```python
from build123d import *

# Parameters (mm, degrees)
F0_W           = 40.7
F0_H           = 23.2
F0_H_2         = 5
F0_H_3         = 1.8
F1_DEPTH       = 10.5
F2_D           = 3
F2_CBORE_D     = 6
F2_CBORE_DEPTH = 5
F3_D           = 3
F3_CBORE_D     = 6
F3_CBORE_DEPTH = 5
F4_DEPTH       = 4
F6_DEPTH       = 8.8
F7_T1_DEPTH    = 13.8
F7_T3_DEPTH    = 20.5
F7_T5_DEPTH    = 33.2
F7_T7_DEPTH    = 50.6498743711
F7_T9_DEPTH    = 50.7
F7_T11_DEPTH   = 5
F8_R           = 0.5
F10_DEPTH      = 2.5
F11_DEPTH      = 1.5


# Not quite as in the source:
# - a fillet or chamfer that OpenCascade refuses, or shapes differently, is made with other operations: its cross-section is extruded or revolved along the edge and cut away or added


with BuildPart() as f1:
    # F0 (on Top) → F1 (new body)
    with BuildSketch(Plane.XY):
        with Locations((0, -3.4)):
            Rectangle(F0_W, F0_H)
        with Locations((0, 10.7)):
            Rectangle(F0_W, F0_H_2)
        with Locations((0, 14.1)):
            Rectangle(F0_W, F0_H_3)
    extrude(amount=F1_DEPTH)

    # F2 (through all)
    with Locations(Plane(origin=(0, 0, 0), x_dir=(1, 0, 0), z_dir=(0, 0, -1))):
        with Locations((-16.15, 10.5)):
            CounterBoreHole(F2_D / 2, F2_CBORE_D / 2, F2_CBORE_DEPTH)

    # F3 (through all)
    with Locations(Plane(origin=(0, 0, 0), x_dir=(1, 0, 0), z_dir=(0, 0, -1))):
        with Locations((16.15, 10.5)):
            CounterBoreHole(F3_D / 2, F3_CBORE_D / 2, F3_CBORE_DEPTH)

    # F0 (on Top) → F4 (cut)
    with BuildSketch(Plane.XY):
        with Locations((0, 10.7)):
            Rectangle(F0_W, F0_H_2)
    extrude(amount=F4_DEPTH, mode=Mode.SUBTRACT)

    # F5 (on face) → F6 (cut)
    with BuildSketch(Plane.XY.offset(10.5)):
        Polygon((-12.85, -3.7), (-12.85, -8.6720474064), (-12.85, -15), (12.85, -15), (12.85, -8.5788490251), (12.886153895, -3.7037077804), (14.5, -3.7156760127), (14.5, 8.1671951339), (-14.5, 8.0755921081), (-14.5, -3.7), align=None)
    extrude(amount=-F6_DEPTH, mode=Mode.SUBTRACT)

    # F7: fillet of radius 2 on 10 edges, made by hand

    # F7_s2 → F7_t1 (cut)
    with BuildSketch(Plane.XY.offset(1.7)):
        with BuildLine():
            ThreePointArc((-14.85, -15), (-13.4357864376, -14.4142135624), (-12.85, -13))
            Line((-12.85, -13), (-12.85, -15))
            Line((-12.85, -15), (-14.85, -15))
        make_face()
        with BuildLine():
            ThreePointArc((14.85, -15), (13.4357864376, -14.4142135624), (12.85, -13))
            Line((12.85, -13), (12.85, -15))
            Line((12.85, -15), (14.85, -15))
        make_face()
    extrude(amount=F7_T1_DEPTH, mode=Mode.SUBTRACT)

    # F7_s4 → F7_t3 (cut)
    with BuildSketch(Plane.XY.offset(-5)):
        with BuildLine():
            ThreePointArc((-18.35, -15), (-19.7642135624, -14.4142135624), (-20.35, -13))
            Line((-20.35, -13), (-20.35, -15))
            Line((-20.35, -15), (-18.35, -15))
        make_face()
        with BuildLine():
            ThreePointArc((18.35, -15), (19.7642135624, -14.4142135624), (20.35, -13))
            Line((20.35, -13), (20.35, -15))
            Line((20.35, -15), (18.35, -15))
        make_face()
    extrude(amount=F7_T3_DEPTH, mode=Mode.SUBTRACT)

    # F7_s6 → F7_t5 (cut)
    with BuildSketch(Plane.XZ.offset(-13.2)):
        with BuildLine():
            ThreePointArc((-18.35, 0), (-19.7642135624, 0.5857864376), (-20.35, 2))
            Line((-20.35, 2), (-20.35, 0))
            Line((-20.35, 0), (-18.35, 0))
        make_face()
        with BuildLine():
            ThreePointArc((18.35, 0), (19.7642135624, 0.5857864376), (20.35, 2))
            Line((20.35, 2), (20.35, 0))
            Line((20.35, 0), (18.35, 0))
        make_face()
    extrude(amount=F7_T5_DEPTH, mode=Mode.SUBTRACT)

    # F7_s8 → F7_t7 (cut)
    with BuildSketch(Plane.YZ.offset(-25.3249371855)):
        with BuildLine():
            ThreePointArc((13.2, 1.9899748742), (13.7167603026, 0.6483340877), (15, 0))
            Line((15, 0), (13.2, 0))
            Line((13.2, 0), (13.2, 1.9899748742))
        make_face()
    extrude(amount=F7_T7_DEPTH, mode=Mode.SUBTRACT)

    # F7_s10 → F7_t9 (cut)
    with BuildSketch(Plane.YZ.offset(-25.35)):
        with BuildLine():
            ThreePointArc((6.2, 0), (7.6142135624, 0.5857864376), (8.2, 2))
            Line((8.2, 2), (8.2, 0))
            Line((8.2, 0), (6.2, 0))
        make_face()
    extrude(amount=F7_T9_DEPTH, mode=Mode.SUBTRACT)

    # F7_s12 → F7_t11 (cut)
    with BuildSketch(Plane.XZ.offset(-13.2)):
        with BuildLine():
            ThreePointArc((20.35, 6), (19.7642135624, 4.5857864376), (18.35, 4))
            Line((18.35, 4), (20.35, 4))
            Line((20.35, 4), (20.35, 6))
        make_face()
        with BuildLine():
            ThreePointArc((-20.35, 6), (-19.7642135624, 4.5857864376), (-18.35, 4))
            Line((-18.35, 4), (-20.35, 4))
            Line((-20.35, 4), (-20.35, 6))
        make_face()
    extrude(amount=F7_T11_DEPTH, mode=Mode.SUBTRACT)

    # F8
    f8_edges = [f1.edges().sort_by_distance(p)[0] for p in [
        (0, -15, 0),
        (0, -15, 1.7),
        (-19.764214, -14.414214, 0.585786),
        (19.764214, -14.414214, 0.585786),
    ]]
    fillet(f8_edges, radius=F8_R)

    # F9 (on face) → F10 (join)
    with BuildSketch(Plane.XY.offset(1.7)):
        with BuildLine():
            Line((12.85, -11.5439696237), (-12.85, -11.5439696237))
            Line((-12.85, -11.5439696237), (-12.85, -13))
            ThreePointArc((-12.85, -13), (-13.0181614416, -13.802725044), (-13.4943674962, -14.4704626873))
            Line((-13.4943674962, -14.4704626873), (13.4943674962, -14.4704626873))
            ThreePointArc((13.4943674962, -14.4704626873), (13.0181614416, -13.802725044), (12.85, -13))
            Line((12.85, -13), (12.85, -11.5439696237))
        make_face()
    extrude(amount=F10_DEPTH)

    # F11 (add): a face of the model
    f11_faces = [f1.faces().sort_by_distance(p)[0] for p in [
        (0, 15, 5.25),
    ]]
    extrude(f11_faces, amount=F11_DEPTH)


solid = f1.part
```
The listing builds one solid part. Answer for the finished solid, in the listing's coordinates (mm). A direction names the side the tool comes from. Give positions to 0.01 mm unless a question says otherwise; leave off trailing zeros. Write each loop counter-clockwise with the first axis right and the second up, starting at its lowest first coordinate (ties: lowest second). Pieces come first, ordered by that corner, then holes. Notation, with made-up numbers: M -31,19 L 22,19 A9 ccw 22,32 Z; hole C -8,-34 d11. An arc over 180 degrees is marked long. Write each question's results on one line, items separated by ' | '.
Q1. Section D-D, the plane y = 1 is taken. Write down the section's boundary in (x, z).
Output values:
outline: M -20.35,2 A2 ccw -18.35,0 L 18.35,0 A2 ccw 20.35,2 L 20.35,10.5 L 14.5,10.5 L 14.5,1.7 L -14.5,1.7 L -14.5,10.5 L -20.35,10.5 Z
Q2. A tool of negligible diameter and unlimited length cuts with its end or side. For faces 1 (the cylindrical face through (17.65, -10.57, 7.79)), 2 (the flat face through (-18, -10, 5)), 3 (the flat face through (0, -4, 0)), 4 (the cylindrical face through (-0.28, 7.6, 0.57)), 5 (the flat face through (14.5, 2, 6)), from which of +Z, -Z, +X, -X, +Y, -Y can it reach the whole face along a straight path? Write none if from no direction.
Output values:
face 1: +Z, -Z | face 2: -Z | face 3: -Z, +X, -X, +Y, -Y | face 4: -Z, +X, -X | face 5: +Z
Q3. For a pull along X with two mould halves and no side action, classify faces 6 (the cylindrical face through (-19.75, -2.99, 0.57)), 7 (the cylindrical face through (-13.45, -14.43, 6.82)), 8 (the flat face through (0, -15, 1)), 9 (the flat face through (0, -13, 4.2)) as released by +X, released by -X, zero draft, split by the parting line, or undercut.
Output values:
face 6: released by -X | face 7: undercut | face 8: zero draft | face 9: undercut
Q4. Section A-A, the plane z = 2.5 is taken. Write down the section's boundary in (x, y), then the cut area to 3 significant figures.
Output values:
outline: M -20.35,-13 A2 ccw -18.35,-15 L -14.85,-15 A2 ccw -13.49,-14.47 L 13.49,-14.47 A2 ccw 14.85,-15 L 18.35,-15 A2 ccw 20.35,-13 L 20.35,8.2 L -20.35,8.2 Z; M -20.35,13.2 L 20.35,13.2 L 20.35,16.5 L -20.35,16.5 Z; hole C -16.15,-10.5 d6; hole M -14.5,-3.7 L -12.85,-3.7 L -12.85,-11.54 L 12.85,-11.54 L 12.85,-8.58 L 12.89,-3.7 L 14.5,-3.72 L 14.5,8.17 L -14.5,8.08 Z; hole C 16.15,-10.5 d6 | area: 461 mm2
Q5. Section B-B, the plane x = -16.15 is taken. Write down the section's boundary in (y, z).
Output values:
outline: M -15,0.5 A0.5 ccw -14.5,0 L -13.5,0 L -13.5,5 L -12,5 L -12,10.5 L -15,10.5 Z; M -9,5 L -7.5,5 L -7.5,0 L 6.2,0 A2 ccw 8.2,2 L 8.2,4 L 13.2,4 L 13.2,1.99 A2 ccw 15,0 L 16.5,0 L 16.5,10.5 L -9,10.5 Z
Q6. Flat-ended cylindrical pins translate along their axes: P1, Ø1.2, axis at x = -3, z = 3, coming from the -Y side; P2, Ø4.5, axis at x = -2, z = 3.5, coming from the -Y side; P3, Ø6, axis at x = 1.5, y = -3, coming from the +Z side; P4, Ø1.8, axis at x = -16.15, y = -10.5, coming from the +Z side. Find the tip coordinate at first contact, or state that the pin passes through.
Output values:
P1: y = -14.47 | P2: y = -15 | P3: z = 1.7 | P4: through
Q7. Section C-C, the plane y = -10.5 is taken. Write down the section's boundary in (x, z), then the cut area to 3 significant figures.
Output values:
outline: M -20.35,2 A2 ccw -19.15,0.17 L -19.15,5 L -17.65,5 L -17.65,10.5 L -20.35,10.5 Z; M -14.65,5 L -13.15,5 L -13.15,0 L 13.15,0 L 13.15,5 L 14.65,5 L 14.65,10.5 L 12.85,10.5 L 12.85,1.7 L -12.85,1.7 L -12.85,10.5 L -14.65,10.5 Z; M 17.65,5 L 19.15,5 L 19.15,0.17 A2 ccw 20.35,2 L 20.35,10.5 L 17.65,10.5 Z | area: 107 mm2
Q8. Consider L1, parallel to Y at x = 16.15, z = 2.05; L2, parallel to X at y = -10.5, z = 7.15; L3, parallel to X at y = -8, z = 5.75. Determine where each line is inside the solid, lowest interval first. Write a range as from..to.
Output values:
L1: -15..-13.5, -7.5..8.2, 13.2..16.5 | L2: -20.35..-17.65, -14.65..-12.85, 12.85..14.65, 17.65..20.35 | L3: -20.35..-12.85, 12.85..20.35
